For this review, use the dimensioned drawing (mm, ordinates from the lowest corner) and the shaded views. A direction names the side the tool comes from. Give positions to 0.01 mm unless a question says otherwise; leave off trailing zeros. Loops run counter-clockwise (first coordinate to the right, second up) from the corner with the lowest first, then second, coordinate; pieces in that order, holes last. Notation, with made-up numbers: M 46.5,45.5 L 90.5,45.5 A17 cw 90.5,57.5 Z; hole C 48,63.5 d1. An arc over 180 degrees is marked long. Return JSON: item names as keys, results as strings.
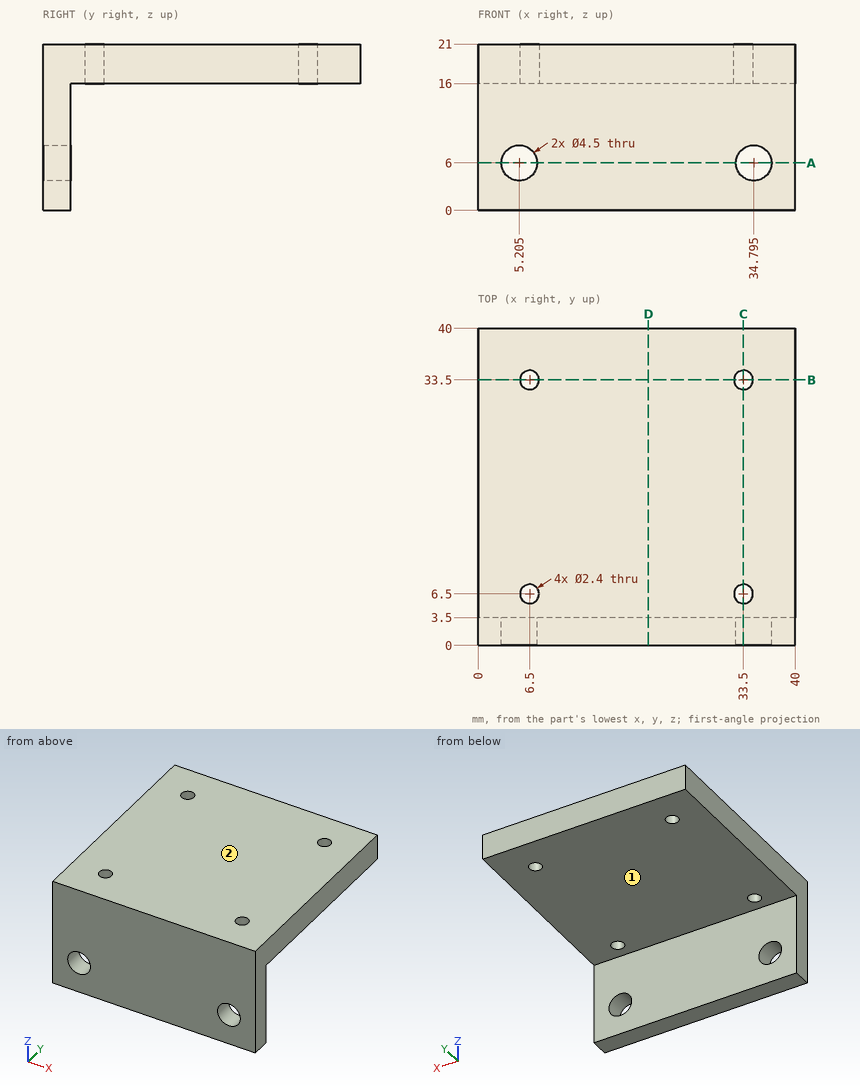
1) Insertion check: pin 1 (12 mm diameter, centred on y = 27, z = 8, fed in from +X); pin 2 (3 mm diameter, centred on x = 33.5, y = 6.5, fed in from -Z); pin 3 (2 mm diameter, centred on x = 35, z = 12, fed in from +Y). Each pin has a flat end and moves straight along its axis. Give the tip position at first contact, or say it passes through.
From the geometry:
{"pin 1": "through", "pin 2": "z = 16", "pin 3": "y = 3.5"}
2) Consider section A-A on z = 6. Write out the cut boundary in (x, y) (3 decimals), then the cut area to 4 significant figures.
From the geometry:
{"outline": "M 0,0 L 2.955,0 L 2.955,3.5 L 0,3.5 Z; M 7.455,0 L 32.545,0 L 32.545,3.5 L 7.455,3.5 Z; M 37.045,0 L 40,0 L 40,3.5 L 37.045,3.5 Z", "area": "108.5 mm²"}
3) Tool access review of the marked faces 1 and 2: name each direction out of +Z, -Z, +X, -X, +Y, -Y from which nothing blocks a thin tool from reaching the whole face with its end or side.
From the geometry:
{"face 1": "-Z, +X, -X, +Y", "face 2": "+Z, +X, -X, +Y, -Y"}
4) Consider section C-C on x = 33.5. Write out the cut boundary in (y, z).
From the geometry:
{"outline": "M 0,0 L 3.5,0 L 3.5,4.16 L 0,4.16 Z; M 0,7.84 L 3.5,7.84 L 3.5,16 L 5.3,16 L 5.3,21 L 0,21 Z; M 7.7,16 L 32.3,16 L 32.3,21 L 7.7,21 Z; M 34.7,16 L 40,16 L 40,21 L 34.7,21 Z"}
5) Wall thickness on L1, parallel to X at y = 1.4, z = 6 (3 decimals); L2, parallel to X at y = 7, z = 18.25; L3, parallel to Z at x = 30.5, y = 35: over which ranges is each line inside the solid? List them lowest first. Write a range as from..to.
From the geometry:
{"L1": "0..2.955, 7.455..32.545, 37.045..40", "L2": "0..5.41, 7.59..32.41, 34.59..40", "L3": "16..21"}
6) Consider section D-D on x = 21.5. Write out the cut boundary in (y, z).
From the geometry:
{"outline": "M 0,0 L 3.5,0 L 3.5,16 L 40,16 L 40,21 L 0,21 Z"}
7) Consider section B-B on y = 33.5. Write out the cut boundary in (x, z), then the cut area to 3 significant figures.
From the geometry:
{"outline": "M 0,16 L 5.3,16 L 5.3,21 L 0,21 Z; M 7.7,16 L 32.3,16 L 32.3,21 L 7.7,21 Z; M 34.7,16 L 40,16 L 40,21 L 34.7,21 Z", "area": "176 mm²"}
